```python
from build123d import *

# Parameters (mm, degrees)
SKETCH1_W           = 195
SKETCH1_H           = 30
BOSS_EXTRUDE1_DEPTH = 8
SKETCH2_W           = 12
SKETCH2_H           = 30
BOSS_EXTRUDE2_DEPTH = 12
SKETCH4_R           = 3.15
CUT_EXTRUDE1_DEPTH  = 199.305320151
FILLET1_R           = 4
FILLET2_R           = 6
BOSS_EXTRUDE4_DEPTH = 30
SKETCH15_W          = 67
SKETCH15_H          = 7
BOSS_EXTRUDE6_DEPTH = 13
SKETCH16_W          = 62
SKETCH16_H          = 6.3
CUT_EXTRUDE4_DEPTH  = 199.408669165
FILLET6_R           = 5
FILLET7_R           = 5
SKETCH17_W          = 10
SKETCH17_H          = 30
BOSS_EXTRUDE7_DEPTH = 6
FILLET8_R           = 3.15
FILLET9_R           = 5
SKETCH20_R          = 3.15
BOSS_EXTRUDE8_DEPTH = 16
SKETCH21_W          = 10
SKETCH21_H          = 30
BOSS_EXTRUDE9_DEPTH = 6
SKETCH22_W          = 10
SKETCH22_H          = 10
CUT_EXTRUDE5_DEPTH  = 6
FILLET10_R          = 5
FILLET11_R          = 3.15


with BuildPart() as part:
    # Sketch1 → Boss-Extrude1 (new body)
    with BuildSketch(Plane(origin=(0, 0, 0), x_dir=(1, 0, 0), z_dir=(0, 1, 0))):
        with Locations((97.5, 15)):
            Rectangle(SKETCH1_W, SKETCH1_H)
    extrude(amount=BOSS_EXTRUDE1_DEPTH)

    # Sketch2 → Boss-Extrude2 (add)
    with BuildSketch(Plane(origin=(0, 8, 0), x_dir=(1, 0, 0), z_dir=(0, 1, 0))):
        with Locations((10.715252385, 15)):
            Rectangle(SKETCH2_W, SKETCH2_H)
    extrude(amount=BOSS_EXTRUDE2_DEPTH)

    # Sketch4 → Cut-Extrude1 (cut, through all)
    with BuildSketch(Plane(origin=(0, 0, -30), x_dir=(-1, 0, 0), z_dir=(0, 0, -1))):
        with Locations((-10.715252385, 14)):
            Circle(SKETCH4_R)
    extrude(amount=-CUT_EXTRUDE1_DEPTH, mode=Mode.SUBTRACT)

    # Fillet1
    fillet1_edges = [part.edges().sort_by_distance(p)[0] for p in [
        (4.715252385, 8, -15),
        (16.715252385, 8, -15),
    ]]
    fillet(fillet1_edges, radius=FILLET1_R)

    # Fillet2
    fillet2_edges = [part.edges().sort_by_distance(p)[0] for p in [
        (4.715252385, 20, -15),
        (16.715252385, 20, -15),
    ]]
    fillet(fillet2_edges, radius=FILLET2_R - 0.0001)  # a hair under: the kernel refuses the full size

    # Sketch11 → Boss-Extrude4 (add)
    with BuildSketch(Plane(origin=(0, 0, -30), x_dir=(-1, 0, 0), z_dir=(0, 0, -1))):
        with BuildLine():
            Line((-16.715252385, 14), (-16.715252385, 12))
            ThreePointArc((-16.715252385, 12), (-17.88682526, 9.171572875), (-20.715252385, 8))
            Line((-20.715252385, 8), (-22.27876013, 8))
            Line((-22.27876013, 8), (-20.715252385, 9))
            ThreePointArc((-20.715252385, 9), (-18.593932042, 9.878679656), (-17.715252385, 12))
            Line((-17.715252385, 12), (-17.715252385, 14))
            ThreePointArc((-17.715252385, 14), (-15.664999853, 18.949747468), (-10.715252385, 21))
            ThreePointArc((-10.715252385, 21), (-5.765504917, 18.949747468), (-3.715252385, 14))
            Line((-3.715252385, 14), (-3.715252385, 12))
            ThreePointArc((-3.715252385, 12), (-2.836572729, 9.878679656), (-0.715252385, 9))
            Line((-0.715252385, 9), (0, 8))
            Line((0, 8), (-0.715252385, 8))
            ThreePointArc((-0.715252385, 8), (-3.54367951, 9.171572875), (-4.715252385, 12))
            Line((-4.715252385, 12), (-4.715252385, 14))
            ThreePointArc((-4.715252385, 14), (-6.472611698, 18.242640687), (-10.715252385, 20))
            ThreePointArc((-10.715252385, 20), (-14.957893072, 18.242640687), (-16.715252385, 14))
        make_face()
    extrude(amount=-BOSS_EXTRUDE4_DEPTH)

    # Sketch15 → Boss-Extrude6 (add)
    with BuildSketch(Plane(origin=(0, 8, 0), x_dir=(1, 0, 0), z_dir=(0, 1, 0))):
        with Locations((161.5, 26.5)):
            Rectangle(SKETCH15_W, SKETCH15_H)
        with Locations((161.5, 3.5)):
            Rectangle(SKETCH15_W, SKETCH15_H)
    extrude(amount=BOSS_EXTRUDE6_DEPTH)

    # Sketch16 → Cut-Extrude4 (cut, through all)
    with BuildSketch(Plane(origin=(0, 0, -30), x_dir=(-1, 0, 0), z_dir=(0, 0, -1))):
        with Locations((-161.5, 15.35)):
            Rectangle(SKETCH16_W, SKETCH16_H)
    extrude(amount=-CUT_EXTRUDE4_DEPTH, mode=Mode.SUBTRACT)

    # Fillet6
    fillet6_edges = [part.edges().sort_by_distance(p)[0] for p in [
        (195, 21, -26.5),
        (128, 21, -26.5),
    ]]
    fillet(fillet6_edges, radius=FILLET6_R)

    # Fillet7
    fillet7_edges = [part.edges().sort_by_distance(p)[0] for p in [
        (128, 8, -26.5),
    ]]
    fillet(fillet7_edges, radius=FILLET7_R)

    # Sketch17 → Boss-Extrude7 (add)
    with BuildSketch(Plane.XZ):
        with Locations((97.5, -15)):
            Rectangle(SKETCH17_W, SKETCH17_H)
    extrude(amount=BOSS_EXTRUDE7_DEPTH)

    # Fillet8
    fillet8_edges = [part.edges().sort_by_distance(p)[0] for p in [
        (192.5, 18.5, -3.5),
        (192.5, 12.2, -3.5),
        (130.5, 18.5, -3.5),
        (130.5, 12.2, -3.5),
    ]]
    fillet(fillet8_edges, radius=FILLET8_R - 0.0001)  # a hair under: the kernel refuses the full size

    # Fillet9
    fillet9_edges = [part.edges().sort_by_distance(p)[0] for p in [
        (128, 8, -3.5),
    ]]
    fillet(fillet9_edges, radius=FILLET9_R)

    # Sketch20 → Boss-Extrude8 (add)
    with BuildSketch(Plane.XY.offset(-23)):
        with BuildLine():
            Line((195, 0), (195, 21))
            Line((195, 21), (128, 21))
            Line((128, 21), (128, 13))
            ThreePointArc((128, 13), (126.535533906, 9.464466094), (123, 8))
            Line((123, 8), (22.27876013, 8))
            Line((22.27876013, 8), (20.715252385, 9))
            ThreePointArc((20.715252385, 9), (18.593932042, 9.878679656), (17.715252385, 12))
            Line((17.715252385, 12), (17.715252385, 14))
            ThreePointArc((17.715252385, 14), (10.715252385, 21), (3.715252385, 14))
            Line((3.715252385, 14), (3.715252385, 12))
            ThreePointArc((3.715252385, 12), (2.836572729, 9.878679656), (0.715252385, 9))
            Line((0.715252385, 9), (0, 8))
            Line((0, 8), (0, 0))
            Line((0, 0), (92.5, 0))
            Line((92.5, 0), (92.5, -6))
            Line((92.5, -6), (102.5, -6))
            Line((102.5, -6), (102.5, 0))
            Line((102.5, 0), (195, 0))
        make_face()
        with Locations(Location((10.715252385, 14, 0), (0, 0, 180))):
            Circle(SKETCH20_R, mode=Mode.SUBTRACT)
        with BuildLine():
            Line((133.65, 12.2), (189.35, 12.2))
            ThreePointArc((189.35, 12.2), (191.577386361, 13.122613639), (192.5, 15.35))
            ThreePointArc((192.5, 15.35), (191.577386361, 17.577386361), (189.35, 18.5))
            Line((189.35, 18.5), (133.65, 18.5))
            ThreePointArc((133.65, 18.5), (131.422613639, 17.577386361), (130.5, 15.35))
            ThreePointArc((130.5, 15.35), (131.422613639, 13.122613639), (133.65, 12.2))
        make_face(mode=Mode.SUBTRACT)
    extrude(amount=BOSS_EXTRUDE8_DEPTH)

    # Sketch21 → Boss-Extrude9 (add)
    with BuildSketch(Plane(origin=(0, 0, 0), x_dir=(-1, 0, 0), z_dir=(0, -1, 0))):
        with Locations((-5, 15)):
            Rectangle(SKETCH21_W, SKETCH21_H)
        with Locations((-190, 15)):
            Rectangle(SKETCH21_W, SKETCH21_H)
    extrude(amount=BOSS_EXTRUDE9_DEPTH)

    # Sketch22 → Cut-Extrude5 (cut)
    with BuildSketch(Plane(origin=(0, -6, 0), x_dir=(-1, 0, 0), z_dir=(0, -1, 0))):
        with Locations((-5, 15)):
            Rectangle(SKETCH22_W, SKETCH22_H)
        with Locations((-97.5, 15)):
            Rectangle(SKETCH22_W, SKETCH22_H)
        with Locations((-190, 15)):
            Rectangle(SKETCH22_W, SKETCH22_H)
    extrude(amount=-CUT_EXTRUDE5_DEPTH, mode=Mode.SUBTRACT)

    # Fillet10
    fillet10_edges = [part.edges().sort_by_distance(p)[0] for p in [
        (128, 21, -11.5),
        (195, 21, -11.5),
    ]]
    fillet(fillet10_edges, radius=FILLET10_R)

    # Fillet11
    fillet11_edges = [part.edges().sort_by_distance(p)[0] for p in [
        (130.5, 18.5, -26.5),
        (130.5, 12.2, -26.5),
        (192.5, 12.2, -26.5),
        (192.5, 18.5, -26.5),
    ]]
    fillet(fillet11_edges, radius=FILLET11_R - 0.0001)  # a hair under: the kernel refuses the full size


solid = part.part
```
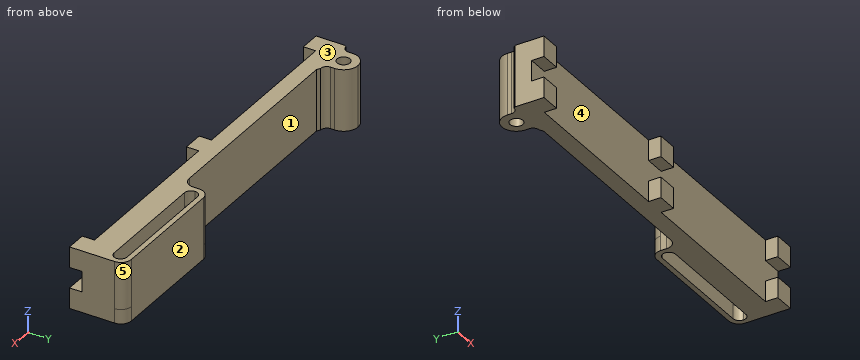
Work out the finished part from the listing and answer in its coordinate system (mm). Face numbers are marked on the shaded views. A direction names the side the tool comes from. Coordinates: 2 decimals unless noted, no trailing zeros. Write each loop counter-clockwise with the first axis right and the second up, starting at its lowest first coordinate (ties: lowest second). Pieces come first, ordered by that corner, then holes. Notation, with made-up numbers: (67, 3.5) - (125, 3.5) arc R5 cw to (125, 11.5) - close; hole circle Ø11 at (49.25, -28). An arc over 180 degrees is marked (long way). Answer as a JSON object with one key per item and string values.
Q1. Find section D-D (x = 50). Write down the section's boundary in (y, z), plus the area to 3 significant figures.
Results list:
{"outline": "(0, -30) - (8, -30) - (8, 0) - (0, 0) - close", "area": "240 mm^2"}
Q2. Which of the six approach directions +Z, -Z, +X, -X, +Y, -Y give full straight-line access (tool end or side, diameter ignored) to the marked faces 1 and 2?
Results list:
{"face 1": "+Z, -Z, +Y", "face 2": "+Z, -Z, +X, -X, +Y"}
Q3. Find section C-C (z = -17.75). Write down the section's boundary in (x, y), plus the area to 3 significant figures.
Results list:
{"outline": "(0, 0) - (195, 0) - (195, 16) arc R5 ccw to (190, 21) - (133, 21) arc R5 ccw to (128, 16) - (128, 13) arc R5 cw to (123, 8) - (22.28, 8) - (20.72, 9) arc R3 cw to (17.72, 12) - (17.72, 14) arc R7 ccw to (3.72, 14) - (3.72, 12) arc R3 cw to (0.72, 9) - (0, 8) - close; hole circle Ø6.3 at (10.72, 14); hole (133.65, 12.2) - (189.35, 12.2) arc R3.15 ccw to (189.35, 18.5) - (133.65, 18.5) arc R3.15 ccw to start", "area": "2,180 mm^2"}
Q4. Consider L1, parallel to X at y = -4.25, z = -28.5; L2, parallel to X at y = 15.5, z = -2.25; L3, parallel to X at y = 13, z = -19.75. Determine where each line is inside the solid, lowest interval first. Write a range as from..to.
Results list:
{"L1": "x = 0..10, 92.5..102.5, 185..195", "L2": "x = 3.88..7.95, 13.49..17.55, 128..130.5, 192.5..195", "L3": "x = 3.72..7.73, 13.7..17.72, 128..131.55, 191.45..195"}
Q5. Find section B-B (y = -2.5). Write down the section's boundary in (x, z).
Results list:
{"outline": "(0, -30) - (10, -30) - (10, -20) - (0, -20) - close; (0, -10) - (10, -10) - (10, 0) - (0, 0) - close; (92.5, -30) - (102.5, -30) - (102.5, -20) - (92.5, -20) - close; (92.5, -10) - (102.5, -10) - (102.5, 0) - (92.5, 0) - close; (185, -30) - (195, -30) - (195, -20) - (185, -20) - close; (185, -10) - (195, -10) - (195, 0) - (185, 0) - close"}
Q6. Find section A-A (x = 164). Write down the section's boundary in (y, z).
Results list:
{"outline": "(0, -30) - (12.2, -30) - (12.2, 0) - (0, 0) - close; (18.5, -30) - (21, -30) - (21, 0) - (18.5, 0) - close"}
Q7. Given pin 1 Ø15 at (x, z) = (130.5, -10.5) entering from -Y; pin 2 Ø3 at (x, z) = (82, -6.5) entering from +Y, each flat-ended and moving along its own axis, determine where each tip first touches the part or whether it passes through.
Results list:
{"pin 1": "stops at y = 0", "pin 2": "stops at y = 8"}
Q8. For a pull along X with two mould halves and no side action, classify the marked faces 3, 4 and 5 as pulls with the +X half, pulls with the -X half, needs draft (parallel to the pull), parting line crosses it, or undercut.
Results list:
{"face 3": "needs draft", "face 4": "undercut", "face 5": "pulls with the +X half"}
